Here's how the part is built. I have some questions about the finished solid (model axes, mm). Round coordinates to 2 decimals unless told otherwise and drop trailing zeros. Write each loop counter-clockwise with the first axis right and the second up, starting at its lowest first coordinate (ties: lowest second). Pieces come first, ordered by that corner, then holes. Notation, with made-up numbers: (86.25, 27) -> (109.25, 27) arc R22 cw to (109.25, 35) -> close; hole circle Ø6 at (45.25, 31.5). An arc over 180 degrees is marked (long way). Answer in a Markdown table with one row per item.
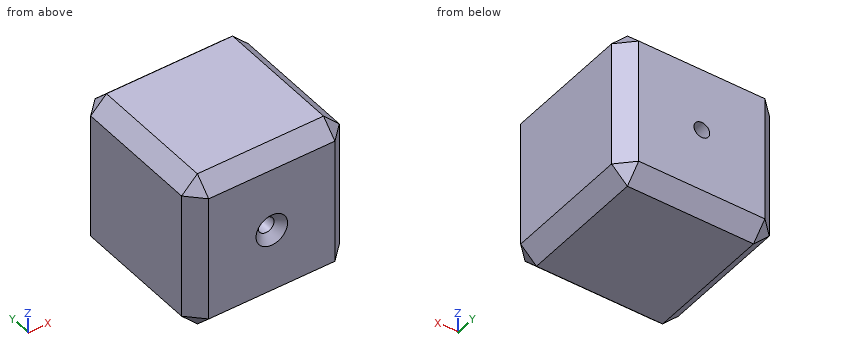
from build123d import *

# Parameters (mm, degrees)
F0_W           = 50
F0_H           = 50
F1_DEPTH       = 50
F2_SIZE        = 5
F4_D           = 5
F4_CSINK_D     = 10
F4_CSINK_ANGLE = 90


with BuildPart() as f1:
    # F0 (on Front) → F1 (new body)
    with BuildSketch(Plane.XZ):
        Rectangle(F0_W, F0_H)
    extrude(amount=F1_DEPTH)

    # F2
    f2_edges = [f1.edges().sort_by_distance(p)[0] for p in [
        (-25, -25, 25),
        (25, -25, 25),
        (0, -50, 25),
        (0, 0, 25),
        (-25, -50, 0),
        (25, -50, 0),
        (0, -50, -25),
        (-25, -25, -25),
        (-25, 0, 0),
        (0, 0, -25),
        (25, 0, 0),
        (25, -25, -25),
    ]]
    chamfer(f2_edges, length=F2_SIZE)

    # F4 (through all)
    with Locations(Plane.XZ.offset(50)):
        with Locations((0, 0)):
            CounterSinkHole(F4_D / 2, F4_CSINK_D / 2, counter_sink_angle=F4_CSINK_ANGLE)


solid = f1.part
1) I want a section at C-C, the plane y = -28.5. List the corners of the cut face in (x, z) for me, and give its area (3 significant figures).
Response:
| item | result |
|---|---|
| outline | (-25, -20) -> (-20, -25) -> (20, -25) -> (25, -20) -> (25, 20) -> (20, 25) -> (-20, 25) -> (-25, 20) -> close; hole circle Ø5 at (0, 0) |
| area | 2,430 mm^2 |
2) I need wall thicknesses on line 1 (X direction, y = -32, z = 0); line 2 (Z direction, x = 21.5, y = -6). Which ranges of each line are inside material? Lowest first, please. Write a range as [from, to].
Response:
| item | result |
|---|---|
| line 1 | x = [-25, -2.5], [2.5, 25] |
| line 2 | z = [-23.5, 23.5] |
3) I want a section at D-D, the plane x = -17.5. List the corners of the cut face in (y, z) for me, and give its area (3 significant figures).
Response:
| item | result |
|---|---|
| outline | (-50, -20) -> (-45, -25) -> (-5, -25) -> (0, -20) -> (0, 20) -> (-5, 25) -> (-45, 25) -> (-50, 20) -> close |
| area | 2,450 mm^2 |
4) I want a section at A-A, the plane z = 0. List the corners of the cut face in (x, y) for me, and give its area (3 significant figures).
Response:
| item | result |
|---|---|
| outline | (-25, -45) -> (-20, -50) -> (-5, -50) -> (-2.5, -47.5) -> (-2.5, 0) -> (-20, 0) -> (-25, -5) -> close; (2.5, -47.5) -> (5, -50) -> (20, -50) -> (25, -45) -> (25, -5) -> (20, 0) -> (2.5, 0) -> close |
| area | 2,190 mm^2 |
5) I want a section at B-B, the plane x = 0. List the corners of the cut face in (y, z) for me.
Response:
| item | result |
|---|---|
| outline | (-50, -20) -> (-45, -25) -> (-5, -25) -> (0, -20) -> (0, -2.5) -> (-47.5, -2.5) -> (-50, -5) -> close; (-50, 5) -> (-47.5, 2.5) -> (0, 2.5) -> (0, 20) -> (-5, 25) -> (-45, 25) -> (-50, 20) -> close |
